Can you work these out from the model? Positions are in its coordinate system, mm. A direction names the side the tool comes from. Give positions to 0.01 mm unless a question says otherwise; leave off trailing zeros. Write each loop counter-clockwise with the first axis right and the second up, starting at its lowest first coordinate (ties: lowest second). Pieces come first, ordered by that corner, then holes. Notation, with made-up numbers: (24.25, 66) -> (82.25, 66) arc R25 ccw to (82.25, 91) -> close; hole circle Ø8 at (-35.5, 71). An arc over 180 degrees is marked (long way). One line per item, written item: value.
from build123d import *

# Parameters (mm, degrees)
F0_R     = 10.65
F0_R_2   = 9.3
F1_DEPTH = 30
F3_DEPTH = 2.5
F4_SIZE  = 0.5
F6_COUNT = 6
F8_ANGLE = 30
F9_COUNT = 6


with BuildPart() as f1:
    # F0 (on Top) → F1 (new body)
    with BuildSketch(Plane.XY):
        Circle(F0_R)
        Circle(F0_R_2, mode=Mode.SUBTRACT)
    extrude(amount=F1_DEPTH)



with BuildPart() as f3:
    # F2 (on Front) → F3 (new body)
    with BuildSketch(Plane.XZ):
        with BuildLine():
            ThreePointArc((0, 3), (1.4142135624, 3.5857864376), (2, 5))
            ThreePointArc((2, 5), (-1.4142135624, 6.4142135624), (0, 3))
        make_face()
    extrude(amount=F3_DEPTH)

    # F4
    f4_edges = [f3.edges().sort_by_distance(p)[0] for p in [
        (0, -2.5, 7),
    ]]
    chamfer(f4_edges, length=F4_SIZE)


with BuildPart() as f3_1:
    # F5: moved
    add(f3.part.moved(Location((0, -9.6, 0))))


with BuildPart() as f6_1:
    # F6: instance of F3
    add(f3_1.part.rotate(Axis((0, 0, 0), (0, 0, -1)), 1 * 360 / F6_COUNT))


with BuildPart() as f6_2:
    # F6: instance of F3
    add(f3_1.part.rotate(Axis((0, 0, 0), (0, 0, -1)), 2 * 360 / F6_COUNT))


with BuildPart() as f6_3:
    # F6: instance of F3
    add(f3_1.part.rotate(Axis((0, 0, 0), (0, 0, -1)), 3 * 360 / F6_COUNT))


with BuildPart() as f6_4:
    # F6: instance of F3
    add(f3_1.part.rotate(Axis((0, 0, 0), (0, 0, -1)), 4 * 360 / F6_COUNT))


with BuildPart() as f6_5:
    # F6: instance of F3
    add(f3_1.part.rotate(Axis((0, 0, 0), (0, 0, -1)), 5 * 360 / F6_COUNT))


with BuildPart() as f7_1:
    # F7: copy of F3
    add(f3_1.part.moved(Location((0, 0, 7))))


with BuildPart() as f7_1_1:
    # F8: moved
    add(f7_1.part.rotate(Axis((0, 0, 0), (0, 0, -1)), F8_ANGLE))


with BuildPart() as f1_1:
    add(f1.part)

    add(f3_1.part)  # F9 merges F3

    add(f6_1.part)  # F9 merges F6_1

    add(f6_2.part)  # F9 merges F6_2

    add(f6_3.part)  # F9 merges F6_3

    add(f6_4.part)  # F9 merges F6_4

    add(f6_5.part)  # F9 merges F6_5

    add(f7_1_1.part)  # F9 merges F7_1
    # F9: F7_1 ×6 about axis
    f9_axis = Axis((0, 0, 0), (0, 0, -1))
    for i in range(1, F9_COUNT):
        add(f7_1_1.part.rotate(f9_axis, i * 360 / F9_COUNT))


solid = f1_1.part
1) Will these pins go through, and if not, where does the flat tip stop? pin 1 (2 mm diameter, centred on x = 0.5, z = 18, fed in from -Y); pin 2 (12 mm diameter, centred on x = -6.5, z = 17.5, fed in from -Y); pin 3 (2 mm diameter, centred on x = 1.5, z = 18, fed in from +Y).
Answer list:
pin 1: stops at y = -10.65
pin 2: stops at y = -11.23
pin 3: stops at y = 10.64
2) I need wall thicknesses on L1, parallel to Y at x = 0, z = 10.25; L2, parallel to X at y = -6.5, z = 18; L3, parallel to X at y = 8.5, z = 17.5. Which ranges of each line are inside material? Lowest first, please.
Answer list:
L1: y = -10.65 to -9.3, 9.3 to 10.65
L2: x = -8.44 to -6.65, 6.65 to 8.44
L3: x = -6.42 to -3.77, 3.77 to 6.42
3) For faces 4 (the face through (-10.49, -6.03, 5.02)), 5 (the face through (-2.3, -10.4, 14.8)), which set-ups out of +Z, -Z, +X, -X, +Y, -Y let a thin tool reach every point of the face, with its end or its side?
Answer list:
face 4: +Z, -Z, -X, -Y
face 5: none
4) If we section it at A-A (z = 18.5): Write out the boundary of the cut face in (x, y).
Answer list:
outline: circle Ø21.3 at (0, 0); hole circle Ø18.6 at (0, 0)
5) We'd pull the mould along X, two halves only. Please class faces 1 (the face through (5, 7.84, 14.79)), 2 (the face through (6.03, -10.49, 12.02)), 3 (the face through (0, -12.1, 5)): released by +X, released by -X, zero draft, split by the parting line, or undercut.
Answer list:
face 1: undercut
face 2: released by +X
face 3: zero draft
